from build123d import *

# Parameters (mm, degrees)
EXTRUDE1_DEPTH = 17
FILLET1_R      = 10
SKETCH2_R      = 2.5
EXTRUDE2_DEPTH = 17
SKETCH3_R      = 2.5
EXTRUDE3_DEPTH = 17


with BuildPart() as part:
    # Sketch1 → Extrude1 (new body)
    with BuildSketch(Plane.XY):
        Polygon((-135.932508131, 32.133218497), (-20.932508131, 32.133218497), (9.067491869, 61.633218497), (54.067491869, 61.633218497), (54.067491869, 54.633218497), (9.067491869, 54.633218497), (-20.932508131, 25.133218497), (-135.932508131, 25.133218497), align=None)
    extrude(amount=EXTRUDE1_DEPTH)

    # Fillet1
    fillet1_edges = [part.edges().sort_by_distance(p)[0] for p in [
        (-20.932508131, 32.133218497, 8.5),
        (9.067491869, 61.633218497, 8.5),
        (9.067491869, 54.633218497, 8.5),
        (-20.932508131, 25.133218497, 8.5),
    ]]
    fillet(fillet1_edges, radius=FILLET1_R)

    # Sketch2 → Extrude2 (cut)
    with BuildSketch(Plane.XZ.offset(-54.633218497)):
        with Locations((44.067491869, 8.5)):
            Circle(SKETCH2_R)
        with Locations((29.067491869, 8.5)):
            Circle(SKETCH2_R)
    extrude(amount=-EXTRUDE2_DEPTH, mode=Mode.SUBTRACT)

    # Sketch3 → Extrude3 (cut)
    with BuildSketch(Plane.XZ.offset(-25.133218497)):
        with Locations((-130.932508131, 8.5)):
            Circle(SKETCH3_R)
    extrude(amount=-EXTRUDE3_DEPTH, mode=Mode.SUBTRACT)


solid = part.part
Here's how the part is built. I have some questions about the finished solid (model axes, mm). A direction names the side the tool comes from. Give positions to 0.01 mm unless a question says otherwise; leave off trailing zeros. Order: outer loops, then holes, each group sorted by start corner. A loop starts at its lowest first (then second) coordinate and runs counter-clockwise, first axis right, second up. Notation, with made-up numbers: (6, -30.75) -> (19, -30.75) arc R23 ccw to (19, -19.75) -> close; hole circle Ø7 at (-31, -39.75). An arc over 180 degrees is marked (long way). One line per item, written item: value. Start each with the question number.
1. Imagine slicing it at B-B, the plane x = -35.5. List the corners of the cut face in (y, z) for me.
2. We'd pull the mould along X, two halves only. Please class faces 3 (the face through (-81, 32.133, 8)), 4 (the face through (54.067, 58, 8)), 5 (the face through (-6.1, 46.72, 8.38)), 6 (the face through (46.377, 58.084, 7.542)): released by +X, released by -X, zero draft, split by the parting line, or undercut.
3. Imagine slicing it at C-C, the plane y = 43. List the corners of the cut face in (x, z) for me.
4. I need wall thicknesses on probe 1 along Y at (x, z) = (15.5, 14.25); probe 2 along Y at (x, z) = (-84, 1.5); probe 3 along X at (y, z) = (27, 10). Which ranges of each line are inside material? Lowest first, please. Write a range as from..to.
5. Imagine slicing it at A-A, the plane z = 8.5. List the corners of the cut face in (x, y) for me, plus the area to 4 significant figures.
6. For faces 1 (the face through (34, 54.633, 8)), 2 (the face through (31.377, 58.084, 7.542)), which set-ups out of +Z, -Z, +X, -X, +Y, -Y let a thin tool reach every point of the face, with its end or its side?
7. Will these pins go through, and if not, where does the flat tip stop? pin 1 Ø6.5 at (x, z) = (44.07, 8.5) entering from -Y; pin 2 Ø6 at (x, z) = (29.07, 8.5) entering from +Y; pin 3 Ø5 at (y, z) = (43.5, 14) entering from -X; pin 4 Ø4 at (x, z) = (9, 6) entering from +Y.
Values follow:
1. outline: (25.13, 0) -> (32.13, 0) -> (32.13, 17) -> (25.13, 17) -> close
2. face 3: zero draft
2. face 4: released by +X
2. face 5: released by -X
2. face 6: undercut
3. outline: (-9.88, 0) -> (-2.76, 0) -> (-2.76, 17) -> (-9.88, 17) -> close
4. probe 1: y = 54.63..61.63
4. probe 2: y = 25.13..32.13
4. probe 3: x = -135.93..-132.93, -128.93..-19.21
5. outline: (-135.93, 25.13) -> (-133.43, 25.13) -> (-133.43, 32.13) -> (-135.93, 32.13) -> close; (-128.43, 25.13) -> (-25.03, 25.13) arc R10 ccw to (-18.01, 28) -> (6.15, 51.76) arc R10 cw to (13.16, 54.63) -> (26.57, 54.63) -> (26.57, 61.63) -> (13.16, 61.63) arc R10 ccw to (6.15, 58.76) -> (-18.01, 35) arc R10 cw to (-25.03, 32.13) -> (-128.43, 32.13) -> close; (31.57, 54.63) -> (41.57, 54.63) -> (41.57, 61.63) -> (31.57, 61.63) -> close; (46.57, 54.63) -> (54.07, 54.63) -> (54.07, 61.63) -> (46.57, 61.63) -> close
5. area: 1,225 mm2
6. face 1: +Z, -Z, +X, -Y
6. face 2: +Y, -Y
7. pin 1: stops at y = 54.63
7. pin 2: stops at y = 61.63
7. pin 3: stops at x = -11.92
7. pin 4: stops at y = 61.4
